```python
from build123d import *

# Parameters (mm, degrees)
SKIZZE1_W                                            = 220
SKIZZE1_H                                            = 60
AUFSATZ_LINEAR_AUSTRAGEN1_DEPTH                      = 8
STIRNSENKUNG_F_R_M4_FLACHKOPFSCHRAUBE_MI_D           = 4.5
STIRNSENKUNG_F_R_M4_FLACHKOPFSCHRAUBE_MI_DEPTH       = 11.5
STIRNSENKUNG_F_R_M4_FLACHKOPFSCHRAUBE_MI_CBORE_D     = 9
STIRNSENKUNG_F_R_M4_FLACHKOPFSCHRAUBE_MI_CBORE_DEPTH = 3.1
STIRNSENKUNG_F_R_M4_FLACHKOPFSCHRAUBE_MI_TIP         = 1.351936393
M3_GEWINDEBOHRUNG1_D                                 = 2.5
M3_GEWINDEBOHRUNG1_DEPTH                             = 8.5
M3_GEWINDEBOHRUNG1_TIP                               = 0.751075774
SKIZZE8_W                                            = 15
SKIZZE8_H                                            = 3
SCHNITT_LINEAR_AUSTRAGEN1_DEPTH                      = 223.18010712
M2_5_GEWINDEBOHRUNG1_D                               = 2.05
M2_5_GEWINDEBOHRUNG1_CSINK_D                         = 2.55
M2_5_GEWINDEBOHRUNG1_CSINK_ANGLE                     = 90


with BuildPart() as part:
    # Skizze1 → Aufsatz-Linear austragen1 (new body)
    with BuildSketch(Plane(origin=(0, 0, 0), x_dir=(1, 0, 0), z_dir=(0, 1, 0))):
        Rectangle(SKIZZE1_W, SKIZZE1_H)
    extrude(amount=AUFSATZ_LINEAR_AUSTRAGEN1_DEPTH)

    # Stirnsenkung für M4 Flachkopfschraube mit Schlitz1
    with Locations(Plane(origin=(0, 8, 0), x_dir=(1, 0, 0), z_dir=(0, 1, 0))):
        with Locations((-102.5, 22.5), (-77.5, 22.5), (-77.5, -2.5), (-102.5, -2.5), (102.5, -2.5), (77.5, -2.5), (77.5, 22.5), (102.5, 22.5)):
            CounterBoreHole(STIRNSENKUNG_F_R_M4_FLACHKOPFSCHRAUBE_MI_D / 2, STIRNSENKUNG_F_R_M4_FLACHKOPFSCHRAUBE_MI_CBORE_D / 2, STIRNSENKUNG_F_R_M4_FLACHKOPFSCHRAUBE_MI_CBORE_DEPTH, depth=STIRNSENKUNG_F_R_M4_FLACHKOPFSCHRAUBE_MI_DEPTH)
            with Locations((0, 0, -(STIRNSENKUNG_F_R_M4_FLACHKOPFSCHRAUBE_MI_DEPTH + STIRNSENKUNG_F_R_M4_FLACHKOPFSCHRAUBE_MI_TIP / 2))):  # 118° drill point
                Cone(0, STIRNSENKUNG_F_R_M4_FLACHKOPFSCHRAUBE_MI_D / 2, STIRNSENKUNG_F_R_M4_FLACHKOPFSCHRAUBE_MI_TIP, mode=Mode.SUBTRACT)

    # M3 Gewindebohrung1
    with Locations(Plane(origin=(0, 8, 0), x_dir=(1, 0, 0), z_dir=(0, 1, 0))):
        with Locations((-50, 12.5), (0, 12.5), (50, 12.5), (100, 12.5), (-100, 12.5), (150, 12.5), (200, 12.5)):
            Hole(M3_GEWINDEBOHRUNG1_D / 2, depth=M3_GEWINDEBOHRUNG1_DEPTH)
            with Locations((0, 0, -(M3_GEWINDEBOHRUNG1_DEPTH + M3_GEWINDEBOHRUNG1_TIP / 2))):  # 118° drill point
                Cone(0, M3_GEWINDEBOHRUNG1_D / 2, M3_GEWINDEBOHRUNG1_TIP, mode=Mode.SUBTRACT)

    # Skizze8 → Schnitt-Linear austragen1 (cut, through all)
    with BuildSketch(Plane.ZY.offset(110)):
        with Locations((17.5, 6.5)):
            Rectangle(SKIZZE8_W, SKIZZE8_H)
    extrude(amount=-SCHNITT_LINEAR_AUSTRAGEN1_DEPTH, mode=Mode.SUBTRACT)

    # M2.5 Gewindebohrung1 (through all)
    with Locations(Plane(origin=(0, 5, 0), x_dir=(1, 0, 0), z_dir=(0, 1, 0))):
        with Locations((-90, -21.5), (0, -21.5), (90, -21.5), (45, -13.5), (-45, -13.5)):
            CounterSinkHole(M2_5_GEWINDEBOHRUNG1_D / 2, M2_5_GEWINDEBOHRUNG1_CSINK_D / 2, counter_sink_angle=M2_5_GEWINDEBOHRUNG1_CSINK_ANGLE)


solid = part.part
```
The listing builds one solid part. Answer for the finished solid, in the listing's coordinates (mm). A direction names the side the tool comes from. Give positions to 0.01 mm unless a question says otherwise; leave off trailing zeros. Order: outer loops, then holes, each group sorted by start corner. A loop starts at its lowest first (then second) coordinate and runs counter-clockwise, first axis right, second up. Notation, with made-up numbers: (86.25, 50.5) -> (144.25, 50.5) arc R20 cw to (144.25, 80.5) -> close; hole circle Ø7 at (35.5, -19). An arc over 180 degrees is marked (long way). One line per item, written item: value.
1) Find section C-C, the plane x = -66.5. Determine the outline of the cut face in (y, z), plus the area to 3 significant figures.
Reported:
outline: (0, -30) -> (8, -30) -> (8, 10) -> (5, 10) -> (5, 25) -> (8, 25) -> (8, 30) -> (0, 30) -> close
area: 435 mm^2
2) Determine the mould class of faces 3 (the cylindrical face through (73.9, 6.5, 5.2)), 4 (the flat face through (-2, 8, -10)), 5 (the flat face through (-110, 4, 0)), 6 (the cylindrical face through (75.42, 2.42, 3.36)) for opening direction X: pulls with the +X half, pulls with the -X half, needs draft (parallel to the pull), parting line crosses it, or undercut.
Reported:
face 3: undercut
face 4: needs draft
face 5: pulls with the -X half
face 6: undercut
3) A tool of negligible diameter and unlimited length cuts with its end or side. For faces 1 (the cylindrical face through (-79.58, 2.42, 3.36)), 2 (the flat face through (100, 4.9, -22)), from which of +Z, -Z, +X, -X, +Y, -Y can it reach the whole face along a straight path? Write none if from no direction.
Reported:
face 1: +Y, -Y
face 2: +Y
4) Find the intervals of material crossed by line 1 (X direction, y = 3.15, z = 13.5) (3 decimals); line 2 (X direction, y = 2.1, z = -22.5); line 3 (Z direction, x = -77.5, y = 6.85), in increasing order.
Reported:
line 1: x = -110 to -46.025, -43.975 to 43.975, 46.025 to 110
line 2: x = -110 to -104.75, -100.25 to -79.75, -75.25 to 75.25, 79.75 to 100.25, 104.75 to 110
line 3: z = -30 to -27, -18 to -2, 7 to 10, 25 to 30
5) Find section B-B, the plane z = 2.5. Count the separate pieces of the cut face and the enclosed holes in it, plus the area to 3 significant figures.
Reported:
separate pieces: 5
enclosed holes: 0
area: 1,560 mm^2
6) Flat-ended cylindrical pins translate along their axes: P1, Ø1.2, axis at x = 45, z = 13.5, coming from the +Y side; P2, Ø10.5, axis at x = -102.5, z = 2.5, coming from the -Y side; P3, Ø5, axis at x = 102.5, z = -22.5, coming from the +Y side. Find the tip coordinate at first contact, or state that the pin passes through.
Reported:
P1: passes through
P2: stops at y = 0
P3: stops at y = 4.9
7) Find section A-A, the plane x = 77.5. Determine the outline of the cut face in (y, z), plus the area to 3 significant figures.
Reported:
outline: (0, -30) -> (8, -30) -> (8, -27) -> (4.9, -27) -> (4.9, -24.75) -> (0, -24.75) -> close; (0, -20.25) -> (4.9, -20.25) -> (4.9, -18) -> (8, -18) -> (8, -2) -> (4.9, -2) -> (4.9, 0.25) -> (0, 0.25) -> close; (0, 4.75) -> (4.9, 4.75) -> (4.9, 7) -> (8, 7) -> (8, 10) -> (5, 10) -> (5, 25) -> (8, 25) -> (8, 30) -> (0, 30) -> close
area: 335 mm^2
